Geometry check sheet. Reference: the model listing, model coordinates, mm. Face numbers are marked on the shaded views. A direction names the side the tool comes from. Round coordinates to 2 decimals unless told otherwise and drop trailing zeros. Order: outer loops, then holes, each group sorted by start corner. A loop starts at its lowest first (then second) coordinate and runs counter-clockwise, first axis right, second up. Notation, with made-up numbers: (86, 73) -> (140, 73) arc R28 ccw to (140, 100) -> close; hole circle Ø8 at (66.5, 75). An arc over 180 degrees is marked (long way). Use a Markdown table: item, result. Add a question column.
Item 1: Sectioned sample at C-C, the plane y = -12.5. Record the cut outline in (x, z).
Item 2: Sectioned sample at A-A, the plane z = 1.75. Record the cut outline in (x, y), and give its area (3 significant figures).
Item 3: Material ranges on probe 1 along Y at (x, z) = (11, 2.25); probe 2 along Z at (x, y) = (-4, 12.5); probe 3 along Y at (x, z) = (-9.5, 4.5), recorded low to high. Write a range as [from, to].
Item 4: Gauge pin test, flat ends, axial feed: pin 1 Ø3.5 at (y, z) = (-12, 2.5) entering from -X; pin 2 Ø2.5 at (y, z) = (-12.5, 2.5) entering from +X; pin 3 Ø2 at (y, z) = (-13, 3) entering from -X; pin 4 Ø10 at (x, y) = (-1, 1) entering from +Z. Record the tip position at first contact, or that the pin passes through.
Item 5: Sectioned sample at B-B, the plane x = -9.5. Record the cut outline in (y, z).
Item 6: Set-up check for the marked faces 1, 2, 3, 4 and 5: record each of +Z, -Z, +X, -X, +Y, -Y from which the full face is reachable in a straight line by a thin tool's end or side.
Item 7: Sectioned sample at D-D, the plane x = 6. Record the cut outline in (y, z), and give its area (3 significant figures).
from build123d import *

# Parameters (mm, degrees)
F0_W     = 40
F0_H     = 28
F1_DEPTH = 1
F2_W     = 13
F2_H     = 3
F3_DEPTH = 7
F4_R     = 2
F2_W_2   = 8.5
F5_DEPTH = 3
F6_R     = 2
F7_DEPTH = 3


with BuildPart() as f1:
    # F0 (on Top) → F1 (new body)
    with BuildSketch(Plane.XY):
        Rectangle(F0_W, F0_H)
    extrude(amount=F1_DEPTH)

    # F2 (on face) → F3 (join)
    with BuildSketch(Plane.XY.offset(1)):
        with Locations((-9.5, -12.5)):
            Rectangle(F2_W, F2_H)
    extrude(amount=F3_DEPTH)

    # F4
    f4_edges = [f1.edges().sort_by_distance(p)[0] for p in [
        (-16, -12.5, 8),
        (-3, -12.5, 8),
    ]]
    fillet(f4_edges, radius=F4_R)

    # F2 (on face) → F5 (join)
    with BuildSketch(Plane.XY.offset(1)):
        with Locations((7.25, -12.5)):
            Rectangle(F2_W_2, F2_H)
    extrude(amount=F5_DEPTH)

    # F6 (on face) → F7 (join)
    with BuildSketch(Plane.XZ.offset(14)):
        with Locations((-9.5, 4.815496)):
            Circle(F6_R)
    extrude(amount=F7_DEPTH)


solid = f1.part
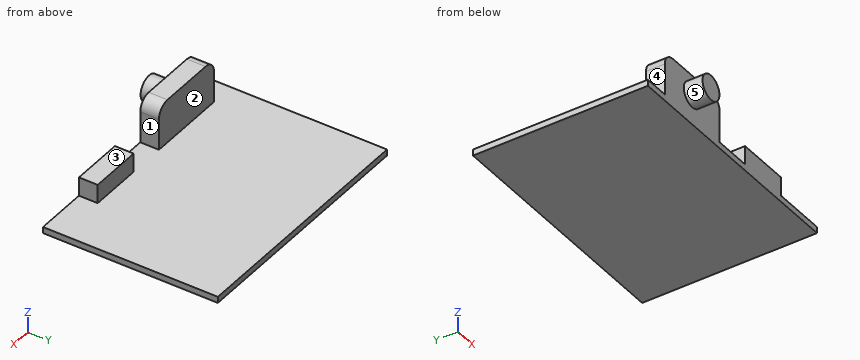
Found:
| question | item | result |
|---|---|---|
| 1 | outline | (-20, 0) -> (20, 0) -> (20, 1) -> (11.5, 1) -> (11.5, 4) -> (3, 4) -> (3, 1) -> (-3, 1) -> (-3, 6) arc R2 ccw to (-5, 8) -> (-14, 8) arc R2 ccw to (-16, 6) -> (-16, 1) -> (-20, 1) -> close |
| 2 | outline | (-16, -14) -> (-3, -14) -> (-3, -11) -> (-16, -11) -> close; (3, -14) -> (11.5, -14) -> (11.5, -11) -> (3, -11) -> close |
| 2 | area | 64.5 mm2 |
| 3 | probe 1 | y = [-14, -11] |
| 3 | probe 2 | z = [0, 1] |
| 3 | probe 3 | y = [-17, -11] |
| 4 | pin 1 | stops at x = -20 |
| 4 | pin 2 | stops at x = 11.5 |
| 4 | pin 3 | stops at x = -16 |
| 4 | pin 4 | stops at z = 1 |
| 5 | outline | (-17, 2.82) -> (-14, 2.82) -> (-14, 0) -> (14, 0) -> (14, 1) -> (-11, 1) -> (-11, 8) -> (-14, 8) -> (-14, 6.82) -> (-17, 6.82) -> close |
| 6 | face 1 | +Z, +Y, -Y |
| 6 | face 2 | +Z, +X, -X, +Y |
| 6 | face 3 | +Z, +X, +Y, -Y |
| 6 | face 4 | +Z, -X, +Y, -Y |
| 6 | face 5 | -Y |
| 7 | outline | (-14, 0) -> (14, 0) -> (14, 1) -> (-11, 1) -> (-11, 4) -> (-14, 4) -> close |
| 7 | area | 37.0 mm2 |
